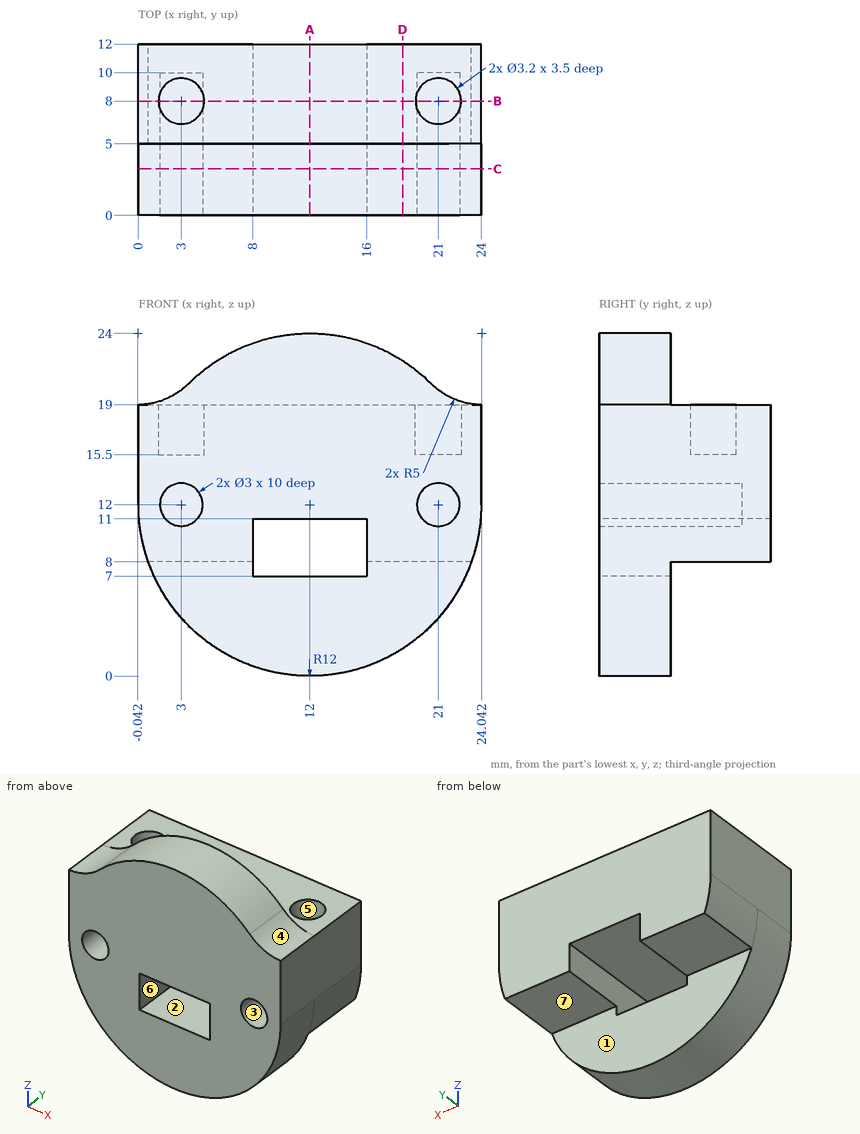
Answer from the drawing. Dimensions are ordinates in mm from the lowest x, y and z of the part. A direction names the side the tool comes from. Coordinates: 2 decimals unless noted, no trailing zeros. Loops run counter-clockwise (first coordinate to the right, second up) from the corner with the lowest first, then second, coordinate; pieces in that order, holes last. Notation, with made-up numbers: (20.5, -32.5) -> (40.5, -32.5) arc R31 ccw to (40.5, -1.5) -> close; hole circle Ø9 at (-13, 47.5). An arc over 180 degrees is marked (long way). Return JSON: item names as keys, results as strings.
Item 1: For a pull along X with two mould halves and no side action, classify the marked faces 4, 5, 6 and 7 as +X half, -X half, draft (parallel to the pull), parting line (faces both ways), or undercut.
Answers:
{"face 4": "+X half", "face 5": "undercut", "face 6": "undercut", "face 7": "draft"}
Item 2: Find section A-A (x = 12). Determine the outline of the cut face in (y, z).
Answers:
{"outline": "(0, 0) -> (5, 0) -> (5, 7) -> (0, 7) -> close; (0, 11) -> (12, 11) -> (12, 19) -> (5, 19) -> (5, 24) -> (0, 24) -> close"}
Item 3: Flat-ended cylindrical pins translate along their axes: P1, Ø2, axis at y = 6, z = 9.5, coming from the -X side; P2, Ø0.9, axis at x = 21.5, z = 12, coming from the -Y side; P3, Ø2.5, axis at x = 11, z = 21, coming from the +Y side. Find the tip coordinate at first contact, or state that the pin passes through.
Answers:
{"P1": "stops at x = 0.09", "P2": "stops at y = 10", "P3": "stops at y = 5"}
Item 4: Find section B-B (y = 8). Determine the outline of the cut face in (x, z).
Answers:
{"outline": "(0, 12) arc R12 ccw to (0.69, 8) -> (8, 8) -> (8, 11) -> (16, 11) -> (16, 8) -> (23.31, 8) arc R12 ccw to (24, 12) -> (24, 19) -> (22.6, 19) -> (22.6, 15.5) -> (19.4, 15.5) -> (19.4, 19) -> (4.6, 19) -> (4.6, 15.5) -> (1.4, 15.5) -> (1.4, 19) -> (0, 19) -> close; hole circle Ø3 at (3, 12); hole circle Ø3 at (21, 12)"}
Item 5: For the marked faces 1, 2 and 3, determine the directions among +Z, -Z, +X, -X, +Y, -Y from which every point of the face is accessible in a straight line to the end or side of a thin tool.
Answers:
{"face 1": "-Z, +X, -X, +Y", "face 2": "+Y, -Y", "face 3": "-Y"}
Item 6: Find section D-D (x = 18.5). Determine the outline of the cut face in (y, z), plus the area to 3 significant figures.
Answers:
{"outline": "(0, 1.91) -> (5, 1.91) -> (5, 8) -> (12, 8) -> (12, 19) -> (5, 19) -> (5, 22.09) -> (0, 22.09) -> close", "area": "178 mm2"}
Item 7: Find section C-C (y = 3.25). Determine the outline of the cut face in (x, z), plus the area to 3 significant figures.
Answers:
{"outline": "(0, 12) arc R12 ccw to (24, 12) -> (24, 19) arc R5 cw to (20.5, 20.47) arc R12 ccw to (3.5, 20.47) arc R5 cw to (0, 19) -> close; hole circle Ø3 at (3, 12); hole (8, 7) -> (16, 7) -> (16, 11) -> (8, 11) -> close; hole circle Ø3 at (21, 12)", "area": "418 mm2"}
Item 8: Find the intervals of material crossed by probe 1 along X at (y, z) = (2.5, 12); probe 2 along X at (y, z) = (4.5, 8) (1 decimal); probe 3 along Y at (x, z) = (3, 17.1), in increasing order.
Answers:
{"probe 1": "x = 0 to 1.5, 4.5 to 19.5, 22.5 to 24", "probe 2": "x = 0.7 to 8, 16 to 23.3", "probe 3": "y = 0 to 6.4, 9.6 to 12"}
